from build123d import *

# Parameters (mm, degrees)
SKETCH1_W                    = 12
SKETCH1_H                    = 35
BASE_FLANGE1_DEPTH           = 2
EDGE_FLANGE1_STRIP_W         = 12
EDGE_FLANGE1_STRIP_H         = 2
EDGE_FLANGE1_STRIP_CUT_DEPTH = 35
EDGE_FLANGE1_DEPTH           = 35
EDGE_FLANGE2_STRIP_W         = 12
EDGE_FLANGE2_STRIP_H         = 2
EDGE_FLANGE2_STRIP_CUT_DEPTH = 35
EDGE_FLANGE2_DEPTH           = 35
EDGE_FLANGE3_STRIP_W         = 12
EDGE_FLANGE3_STRIP_H         = 2
EDGE_FLANGE3_STRIP_CUT_DEPTH = 35
EDGE_FLANGE3_DEPTH           = 35
EDGE_FLANGE4_STRIP_W         = 12
EDGE_FLANGE4_STRIP_H         = 2
EDGE_FLANGE4_STRIP_CUT_DEPTH = 35
EDGE_FLANGE4_DEPTH           = 35
SKETCH18_W                   = 30
SKETCH18_H                   = 14
CUT_EXTRUDE1_DEPTH           = 4
SKETCH19_R                   = 2
CUT_EXTRUDE2_DEPTH           = 49.231213959
SKETCH20_R                   = 2
CUT_EXTRUDE4_DEPTH           = 49.931073971


# Sheet-metal steps are written as plain solids
with BuildPart() as part:
    # Sketch1 → Base-Flange1 (new body)
    with BuildSketch(Plane(origin=(0, 0, 0), x_dir=(1, 0, 0), z_dir=(0, 1, 0))):
        Rectangle(SKETCH1_W, SKETCH1_H)
    extrude(amount=-BASE_FLANGE1_DEPTH)

    # Edge-Flange1 strip (across the edge) → Edge-Flange1 strip cut (cut)
    with BuildSketch(Plane(origin=(6, 0, 17.5), x_dir=(-1, 0, 0), z_dir=(0, 0, -1))):
        with Locations((-2, -1)):
            Rectangle(EDGE_FLANGE1_STRIP_W, EDGE_FLANGE1_STRIP_H)
    extrude(amount=EDGE_FLANGE1_STRIP_CUT_DEPTH, mode=Mode.SUBTRACT)

    # Edge-Flange1 section (across the edge) → Edge-Flange1 (add)
    with BuildSketch(Plane(origin=(6, 0, 17.5), x_dir=(-1, 0, 0), z_dir=(0, 0, -1))):
        with BuildLine():
            Line((0, 2), (0, 16))
            Line((0, 16), (2, 16))
            Line((2, 16), (2, 2))
            ThreePointArc((2, 2), (2.585786438, 0.585786438), (4, 0))
            Line((4, 0), (4, -2))
            ThreePointArc((4, -2), (1.171572875, -0.828427125), (0, 2))
        make_face()
    extrude(amount=EDGE_FLANGE1_DEPTH)

    # Edge-Flange2 strip (across the edge) → Edge-Flange2 strip cut (cut)
    with BuildSketch(Plane(origin=(6, 16, -17.5), x_dir=(0, -1, 0), z_dir=(0, 0, 1))):
        with Locations((-2, -1)):
            Rectangle(EDGE_FLANGE2_STRIP_W, EDGE_FLANGE2_STRIP_H)
    extrude(amount=EDGE_FLANGE2_STRIP_CUT_DEPTH, mode=Mode.SUBTRACT)

    # Edge-Flange2 section (across the edge) → Edge-Flange2 (add)
    with BuildSketch(Plane(origin=(6, 16, -17.5), x_dir=(0, -1, 0), z_dir=(0, 0, 1))):
        with BuildLine():
            Line((0, 2), (0, 24))
            Line((0, 24), (2, 24))
            Line((2, 24), (2, 2))
            ThreePointArc((2, 2), (2.585786438, 0.585786438), (4, 0))
            Line((4, 0), (4, -2))
            ThreePointArc((4, -2), (1.171572875, -0.828427125), (0, 2))
        make_face()
    extrude(amount=EDGE_FLANGE2_DEPTH)

    # Edge-Flange3 strip (across the edge) → Edge-Flange3 strip cut (cut)
    with BuildSketch(Plane(origin=(30, 14, -17.5), x_dir=(-1, 0, 0), z_dir=(0, 0, 1))):
        with Locations((-2, -1)):
            Rectangle(EDGE_FLANGE3_STRIP_W, EDGE_FLANGE3_STRIP_H)
    extrude(amount=EDGE_FLANGE3_STRIP_CUT_DEPTH, mode=Mode.SUBTRACT)

    # Edge-Flange3 section (across the edge) → Edge-Flange3 (add)
    with BuildSketch(Plane(origin=(30, 14, -17.5), x_dir=(-1, 0, 0), z_dir=(0, 0, 1))):
        with BuildLine():
            Line((0, 2), (0, 16))
            Line((0, 16), (2, 16))
            Line((2, 16), (2, 2))
            ThreePointArc((2, 2), (2.585786438, 0.585786438), (4, 0))
            Line((4, 0), (4, -2))
            ThreePointArc((4, -2), (1.171572875, -0.828427125), (0, 2))
        make_face()
    extrude(amount=EDGE_FLANGE3_DEPTH)

    # Edge-Flange4 strip (across the edge) → Edge-Flange4 strip cut (cut)
    with BuildSketch(Plane(origin=(30, -2, 17.5), x_dir=(0, 1, 0), z_dir=(0, 0, -1))):
        with Locations((-2, -1)):
            Rectangle(EDGE_FLANGE4_STRIP_W, EDGE_FLANGE4_STRIP_H)
    extrude(amount=EDGE_FLANGE4_STRIP_CUT_DEPTH, mode=Mode.SUBTRACT)

    # Edge-Flange4 section (across the edge) → Edge-Flange4 (add)
    with BuildSketch(Plane(origin=(30, -2, 17.5), x_dir=(0, 1, 0), z_dir=(0, 0, -1))):
        with BuildLine():
            Line((0, 2), (0, 12))
            Line((0, 12), (2, 12))
            Line((2, 12), (2, 2))
            ThreePointArc((2, 2), (2.585786438, 0.585786438), (4, 0))
            Line((4, 0), (4, -2))
            ThreePointArc((4, -2), (1.171572875, -0.828427125), (0, 2))
        make_face()
    extrude(amount=EDGE_FLANGE4_DEPTH)

    # Sketch18 → Cut-Extrude1 (cut)
    with BuildSketch(Plane(origin=(0, 16, 0), x_dir=(1, 0, 0), z_dir=(0, 1, 0))):
        with Locations((17, -10.5)):
            Rectangle(SKETCH18_W, SKETCH18_H)
    extrude(amount=-CUT_EXTRUDE1_DEPTH, mode=Mode.SUBTRACT)

    # Sketch19 → Cut-Extrude2 (cut, through all)
    with BuildSketch(Plane(origin=(0, 0, 0), x_dir=(1, 0, 0), z_dir=(0, 1, 0))):
        with Locations(Location((-2, 12.5, 0), (0, 0, 270))):
            Circle(SKETCH19_R)
        with Locations(Location((-2, -12.5, 0), (0, 0, 270))):
            Circle(SKETCH19_R)
        with Locations(Location((36, 12.5, 0), (0, 0, 270))):
            Circle(SKETCH19_R)
        with Locations(Location((36, -12.5, 0), (0, 0, 270))):
            Circle(SKETCH19_R)
    extrude(amount=-CUT_EXTRUDE2_DEPTH, mode=Mode.SUBTRACT)

    # Sketch20 → Cut-Extrude4 (cut, through all)
    with BuildSketch(Plane(origin=(0, 16, 0), x_dir=(1, 0, 0), z_dir=(0, 1, 0))):
        with Locations(Location((17, 9.5, 0), (0, 0, 270))):
            Circle(SKETCH20_R)
        with Locations(Location((17, 1.5, 0), (0, 0, 270))):
            Circle(SKETCH20_R)
    extrude(amount=-CUT_EXTRUDE4_DEPTH, mode=Mode.SUBTRACT)


solid = part.part
For this review, take the finished solid that the model builds, in its own axes (mm). A direction names the side the tool comes from. Coordinates: 2 decimals unless noted, no trailing zeros. Order: outer loops, then holes, each group sorted by start corner. A loop starts at its lowest first (then second) coordinate and runs counter-clockwise, first axis right, second up. Notation, with made-up numbers: (17, 65.5) - (43, 65.5) arc R25 ccw to (43, 89.5) - close; hole circle Ø7 at (-30.75, 29). An arc over 180 degrees is marked (long way). Answer as CSV lines item,"result". Start each with the question number.
1) To check wall thickness, follow line 1 along X through (y, z) = (9.25, 9.5); line 2 along X through (y, z) = (-0.55, -12.5); line 3 along X through (y, z) = (-0.6, -12.5). State the ranges of each line that lie inside material, in increasing order. Write a range as [from, to].
2) Add section C-C (y = 3.5). State the section outline as (x, z) points.
3) Add section B-B (z = -1.5). State the section outline as (x, y) points, then the cut area to 3 significant figures.
4) Add section D-D (z = -12.5). State the section outline as (x, y) points, then the cut area to 3 significant figures.
5) Draft analysis for pull direction X (two halves, no side actions). For faces 4 (the flat face through (28, 7, 0)), 5 (the flat face through (30, 7, 0)), 6 (the flat face through (18.1, 14.4, -17.5)), state which applies: +X half, -X half, draft (parallel to the pull), parting line (faces both ways), or undercut.
6) Add section A-A (x = -2). State the section outline as (y, z) points, then the cut area to 3 significant figures.
7) Insertion check: P1, Ø6.5, axis at x = 36, z = -12.5, coming from the +Y side; P2, Ø3, axis at x = 17, z = -1.5, coming from the +Y side; P3, Ø1.6, axis at x = 5, z = 10, coming from the +Y side; P4, Ø1.2, axis at x = 14.5, y = 14.5, coming from the +Z side. Each pin has a flat end and moves straight along its axis. Give the tip position at first contact, or say it passes through.
8) Machinability: for faces 1 (the cylindrical face through (28.797, 14.859, -7.147)), 2 (the flat face through (5, 12, 10)), 3 (the cylindrical face through (29.141, -0.797, 0.245)), which of the approach directions +Z, -Z, +X, -X, +Y, -Y give a long, thin tool a straight path to every point of the face, cutting with its end or side? Answer none if there is none.
Result:
1,line 1,"[4, 6], [28, 30]"
1,line 2,"[-6, -4], [0, 5.08], [28.92, 34], [38, 42]"
1,line 3,"[-6, -4], [0, 5.04], [28.96, 34], [38, 42]"
2,outline,"(4, -17.5) - (6, -17.5) - (6, 17.5) - (4, 17.5) - close; (28, -17.5) - (30, -17.5) - (30, 17.5) - (28, 17.5) - close"
3,outline,"(-6, -2) - (2, -2) arc R4 ccw to (6, 2) - (6, 12) arc R2 cw to (8, 14) - (15, 14) - (15, 16) - (8, 16) arc R4 ccw to (4, 12) - (4, 2) arc R2 cw to (2, 0) - (-6, 0) - close; (19, 14) - (26, 14) arc R2 cw to (28, 12) - (28, 2) arc R4 ccw to (32, -2) - (42, -2) - (42, 0) - (32, 0) arc R2 cw to (30, 2) - (30, 12) arc R4 ccw to (26, 16) - (19, 16) - close"
3,area,"142 mm^2"
4,outline,"(-6, -2) - (-4, -2) - (-4, 0) - (-6, 0) - close; (0, -2) - (2, -2) arc R4 ccw to (6, 2) - (6, 12) arc R2 cw to (8, 14) - (26, 14) arc R2 cw to (28, 12) - (28, 2) arc R4 ccw to (32, -2) - (34, -2) - (34, 0) - (32, 0) arc R2 cw to (30, 2) - (30, 12) arc R4 ccw to (26, 16) - (8, 16) arc R4 ccw to (4, 12) - (4, 2) arc R2 cw to (2, 0) - (0, 0) - close; (38, -2) - (42, -2) - (42, 0) - (38, 0) - close"
4,area,"134 mm^2"
5,face 4,"undercut"
5,face 5,"+X half"
5,face 6,"draft"
6,outline,"(-2, -17.5) - (0, -17.5) - (0, -14.5) - (-2, -14.5) - close; (-2, -10.5) - (0, -10.5) - (0, 10.5) - (-2, 10.5) - close; (-2, 14.5) - (0, 14.5) - (0, 17.5) - (-2, 17.5) - close"
6,area,"54.0 mm^2"
7,P1,"y = 0"
7,P2,"through"
7,P3,"y = 12"
7,P4,"z = 3.5"
8,face 1,"+Z, -Z, +X, +Y"
8,face 2,"+Z, +X, -X, +Y"
8,face 3,"+Z, -Z, -Y"
